```python
from build123d import *

# Parameters (mm, degrees)
F1_DEPTH = 12.7
F2_SIZE  = 3.302
F3_SIZE  = 0.0508


with BuildPart() as f1:
    # F0 (on Front) → F1 (new body)
    with BuildSketch(Plane.XZ):
        with BuildLine():
            Line((77.7875, -15.875), (77.7875, 15.875))
            Line((77.7875, 15.875), (60.3377, 15.875))
            Line((60.3377, 15.875), (60.231681, 0))
            ThreePointArc((60.231681, 0), (54.9402, -5.291481), (49.648719, 0))
            Line((49.648719, 0), (49.53, 0))
            Line((49.53, 0), (49.53, 15.875))
            Line((49.53, 15.875), (-77.7875, 15.875))
            Line((-77.7875, 15.875), (-77.7875, -15.875))
            Line((-77.7875, -15.875), (77.7875, -15.875))
        make_face()
        with BuildLine():
            Line((2.8702, -6.7564), (-54.9402, -6.7564))
            ThreePointArc((-54.9402, -6.7564), (-61.6966, 0), (-54.9402, 6.7564))
            Line((-54.9402, 6.7564), (2.8702, 6.7564))
            ThreePointArc((2.8702, 6.7564), (9.6266, 0), (2.8702, -6.7564))
        make_face(mode=Mode.SUBTRACT)
    extrude(amount=F1_DEPTH)

    # F2
    f2_edges = [f1.edges().sort_by_distance(p)[0] for p in [
        (-77.7875, -6.35, 15.875),
        (-77.7875, -6.35, -15.875),
        (77.7875, -6.35, -15.875),
        (77.7875, -6.35, 15.875),
    ]]
    chamfer(f2_edges, length=F2_SIZE)

    # F3
    f3_edges = [f1.edges().sort_by_distance(p)[0] for p in [
        (-26.035, -12.7, 6.7564),
        (-61.6966, -12.7, 0),
        (-26.035, -12.7, -6.7564),
        (9.6266, -12.7, 0),
        (-61.6966, 0, 0),
        (-26.035, 0, -6.7564),
        (-26.035, 0, 6.7564),
        (9.6266, 0, 0),
    ]]
    chamfer(f3_edges, length=F3_SIZE)


solid = f1.part
```
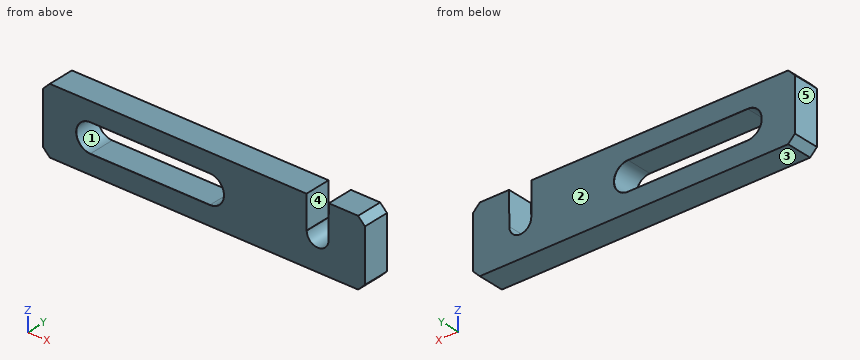
Input: part model. Units: mm. Frame: model coordinates. Face numbers are marked on the shaded views. A direction names the side the tool comes from. Round coordinates to 2 decimals unless told otherwise and drop trailing zeros. Write each loop counter-clockwise with the first axis right and the second up, starting at its lowest first coordinate (ties: lowest second). Pieces come first, ordered by that corner, then holes. Notation, with made-up numbers: M 9.5,-25.5 L 55.5,-25.5 A5 ccw 55.5,-21.5 Z; hole C 80.25,-37.5 d5. An arc over 180 degrees is marked long. Write each question's results on one line, items separated by ' | '.
Q1. Line query: line 1 along Z through (x, y) = (0, -10.25) (3 decimals); line 2 along X through (y, z) = (-0.75, 12); line 3 along X through (y, z) = (-6.5, 3.5). Output: solid intervals per line, ascending.
Results:
line 1: z = -15.875 to -6.756, 6.756 to 15.875 | line 2: x = -77.79 to 49.53, 60.31 to 77.79 | line 3: x = -77.79 to -60.72, 8.65 to 49.53, 60.26 to 77.79
Q2. Draft query along X for the marked faces 3, 4 and 5. Return one class per face: released by +X, released by -X, zero draft, split by the parting line, or undercut.
Results:
face 3: zero draft | face 4: undercut | face 5: released by -X
Q3. Pin query (flat end, axial travel): P1, Ø1, axis at x = -56, z = -4.5, coming from the +Y side. Return the tip coordinate at first contact, or that it passes through.
Results:
P1: passes through
Q4. Section query C-C (z = -2). State how many separate pieces and enclosed holes the cut face has, and give its area (3 significant figures).
Results:
separate pieces: 3 | enclosed holes: 0 | area: 953 mm^2
Q5. Section query B-B (x = -29). Return loops of the section in (y, z) (3 decimals).
Results:
outline: M -12.7,-15.875 L 0,-15.875 L 0,-6.807 L -0.051,-6.756 L -12.649,-6.756 L -12.7,-6.807 Z; M -12.7,6.807 L -12.649,6.756 L -0.051,6.756 L 0,6.807 L 0,15.875 L -12.7,15.875 Z
Q6. Access query for the marked faces 1 and 2. Directions: +Z, -Z, +X, -X, +Y, -Y. A direction counts if a zero-diameter tool reaches every point of the face in a straight line with its end or side. Return the directions, or none.
Results:
face 1: +Y, -Y | face 2: +Z, -Z, +X, -X, +Y
